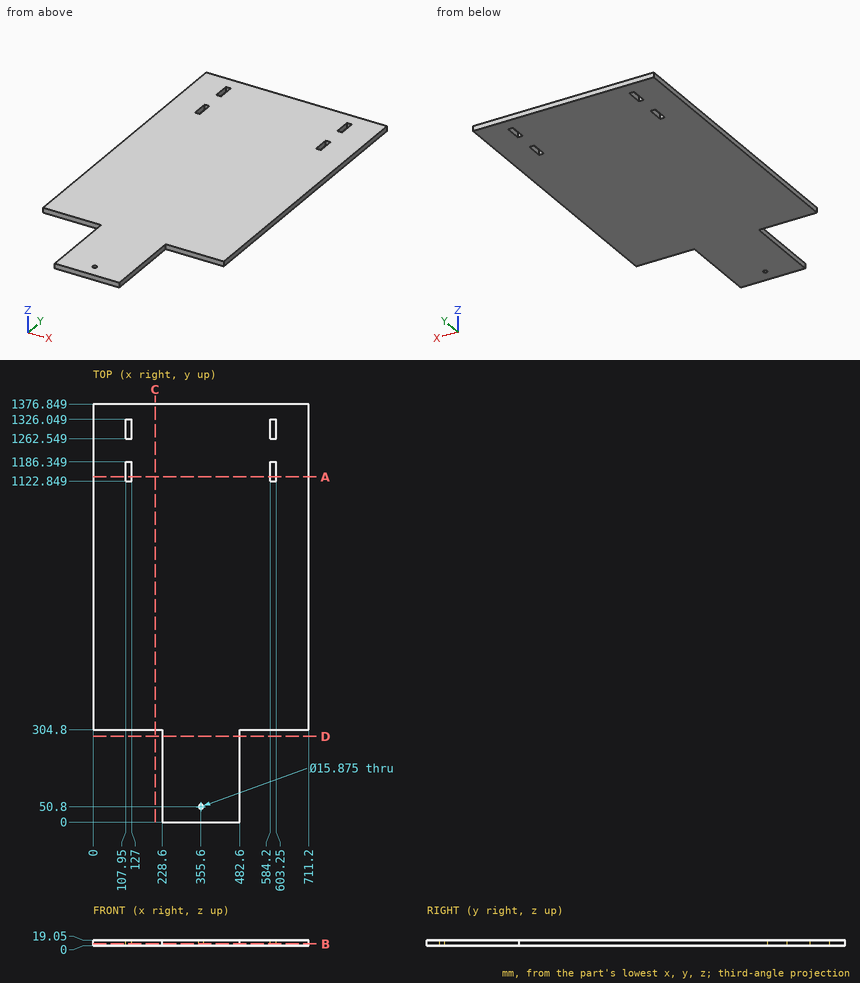
Study the drawing (mm; zero at the part's minimum x, y, z) and answer. Coordinates: 2 decimals unless noted, no trailing zeros. Write each loop counter-clockwise with the first axis right and the second up, starting at its lowest first coordinate (ties: lowest second). Pieces come first, ordered by that corner, then holes. Notation, with made-up numbers: (61, -9) - (75, -9) arc R22 cw to (75, 6) - close; hole circle Ø5 at (64, 44). An arc over 180 degrees is marked (long way). Return JSON: item names as keys, results as strings. Group by question number.
1. A cutting plane is placed at A-A, the plane y = 1137. Determine the outline of the cut face in (x, z).
2. A cutting plane is placed at D-D, the plane y = 282.5. Determine the outline of the cut face in (x, z).
3. Straight lines are drawn through the part: L1, parallel to Y at x = 593.5, z = 6.5; L2, parallel to Y at x = 355.6, z = 14.75; L3, parallel to Y at x = 530, z = 9.25. For each, find the intervals that lie inside material, in ascending order.
4. A cutting plane is placed at C-C, the plane x = 205. Determine the outline of the cut face in (y, z), plus the area to 3 significant figures.
5. A cutting plane is placed at B-B, the plane z = 6.25. Give the number of separate pieces and of enclosed holes in the cut face, plus the area to 3 significant figures.
6. Given pin 1 (9.5 mm diameter, centred on x = 121, z = 13.5, fed in from -Y), flat-ended and moving along its own axis, determine where the tip first touches the part or whether it passes through.
Ans:
{
 "1": {"outline": "(0, 0) - (107.95, 0) - (107.95, 19.05) - (0, 19.05) - close; (127, 0) - (584.2, 0) - (584.2, 19.05) - (127, 19.05) - close; (603.25, 0) - (711.2, 0) - (711.2, 19.05) - (603.25, 19.05) - close"},
 "2": {"outline": "(228.6, 0) - (482.6, 0) - (482.6, 19.05) - (228.6, 19.05) - close"},
 "3": {"L1": "304.8 to 1122.85, 1186.35 to 1262.55, 1326.05 to 1376.85", "L2": "0 to 42.86, 58.74 to 1376.85", "L3": "304.8 to 1376.85"},
 "4": {"outline": "(304.8, 0) - (1376.85, 0) - (1376.85, 19.05) - (304.8, 19.05) - close", "area": "20,400 mm²"},
 "5": {"separate pieces": "1", "enclosed holes": "5", "area": "835,000 mm²"},
 "6": {"pin 1": "y = 304.8"}
}
